```python
from build123d import *

# Parameters (mm, degrees)
ESQUISSE2_R             = 1.5
ENL_V_MAT_EXTRU_1_DEPTH = 14.57387196


with BuildPart() as part:
    # Esquisse1 → Révolution1 (revolve)
    with BuildSketch(Plane.XY, mode=Mode.PRIVATE) as r_volution1_sk:
        Polygon((2.5, 0), (8, 0), (8, 2.5), (3.5, 2.5), (3.5, 7.5), (2.5, 7.5), align=None)
    revolve(r_volution1_sk.sketch.rotate(Axis((0, 0, 0), (0, 1, 0)), 90), axis=Axis((0, 0, 0), (0, 1, 0)))

    # Esquisse2 → Enlèv. mat.-Extru.1 (cut, through all)
    with BuildSketch(Plane.XZ):
        with Locations(Location((0, 6, 0), (0, 0, 270))):
            Circle(ESQUISSE2_R)
        with Locations(Location((5.196152423, -3, 0), (0, 0, 270))):
            Circle(ESQUISSE2_R)
        with Locations(Location((-5.196152423, -3, 0), (0, 0, 270))):
            Circle(ESQUISSE2_R)
    extrude(amount=-ENL_V_MAT_EXTRU_1_DEPTH, mode=Mode.SUBTRACT)


solid = part.part
```
Part model, mm, in its own coordinate system. A direction names the side the tool comes from. Coordinates: 2 decimals unless noted, no trailing zeros. Order: outer loops, then holes, each group sorted by start corner. A loop starts at its lowest first (then second) coordinate and runs counter-clockwise, first axis right, second up. Notation, with made-up numbers: (75.5, 40.5) - (113.5, 40.5) arc R18 ccw to (113.5, 50.5) - close; hole circle Ø8 at (40, 3). An arc over 180 degrees is marked (long way). Return JSON: item names as keys, results as strings. Group by question number.
Item 1: Drill centre lines: probe 1 along X at (y, z) = (4, 0); probe 2 along X at (y, z) = (1.9, -3); probe 3 along Y at (x, z) = (5.5, 3.25). Where is each one in solid material? Low to high. Write a range as from..to.
Item 2: Cut at C-C (z = -2.25). List the corners of the cut face in (x, y).
Item 3: Pin check, flat tips, straight feed: pin 1 (2 mm diameter, centred on x = -3.5, z = 5.5, fed in from +Y); pin 2 (3 mm diameter, centred on y = 3.5, z = 5.5, fed in from -X); pin 3 (4 mm diameter, centred on x = 3, y = 3, fed in from +Z). Stop position of each tip, or through.
Item 4: Cut at A-A (z = 0). List the corners of the cut face in (x, y), plus the area to 3 significant figures.
Item 5: Cut at B-B (x = 0). List the corners of the cut face in (y, z), plus the area to 3 significant figures.
Item 6: Cut at D-D (x = 5.5). List the corners of the cut face in (y, z).
Item 7: Pull direction Z, two halves, no side cores. Call faces 1 (the face through (3.105, 5.035, -1.615)), 2 (the face through (2, 7.5, -2)), 3 (the face through (0.07, 1.23, 7.5)): pulls with the +Z half, pulls with the -Z half, needs draft (parallel to the pull), parting line crosses it, or undercut.
Item 8: Which spindle directions (+Z, -Z, +X, -X, +Y, -Y) get a long thin tool onto all of the face, cutting with end or side? Do faces 4 (the face through (1.7, 2.5, -3.4)), 5 (the face through (-0.1, 3.7, 2.5)). Say none if no direction does.
Check values:
{
 "1": {"probe 1": "x = -3.5..-2.5, 2.5..3.5", "probe 2": "x = -7.42..-6.7, -3.7..3.7, 6.7..7.42", "probe 3": "y = 0..2.5"},
 "2": {"outline": "(-7.68, 0) - (-6.5, 0) - (-6.5, 2.5) - (-7.68, 2.5) - close; (-3.9, 0) - (-1.09, 0) - (-1.09, 7.5) - (-2.68, 7.5) - (-2.68, 2.5) - (-3.9, 2.5) - close; (1.09, 0) - (3.9, 0) - (3.9, 2.5) - (2.68, 2.5) - (2.68, 7.5) - (1.09, 7.5) - close; (6.5, 0) - (7.68, 0) - (7.68, 2.5) - (6.5, 2.5) - close"},
 "3": {"pin 1": "stops at y = 2.5", "pin 2": "stops at x = -6.69", "pin 3": "stops at z = 7.93"},
 "4": {"outline": "(-8, 0) - (-2.5, 0) - (-2.5, 7.5) - (-3.5, 7.5) - (-3.5, 2.5) - (-8, 2.5) - close; (2.5, 0) - (8, 0) - (8, 2.5) - (3.5, 2.5) - (3.5, 7.5) - (2.5, 7.5) - close", "area": "37.5 mm2"},
 "5": {"outline": "(0, -8) - (2.5, -8) - (2.5, -3.5) - (7.5, -3.5) - (7.5, -2.5) - (0, -2.5) - close; (0, 2.5) - (7.5, 2.5) - (7.5, 3.5) - (2.5, 3.5) - (2.5, 4.5) - (0, 4.5) - close; (0, 7.5) - (2.5, 7.5) - (2.5, 8) - (0, 8) - close", "area": "30.0 mm2"},
 "6": {"outline": "(0, -5.81) - (2.5, -5.81) - (2.5, -4.47) - (0, -4.47) - close; (0, -1.53) - (2.5, -1.53) - (2.5, 5.81) - (0, 5.81) - close"},
 "7": {"face 1": "parting line crosses it", "face 2": "needs draft", "face 3": "undercut"},
 "8": {"face 4": "+Y", "face 5": "+Y, -Y"}
}
